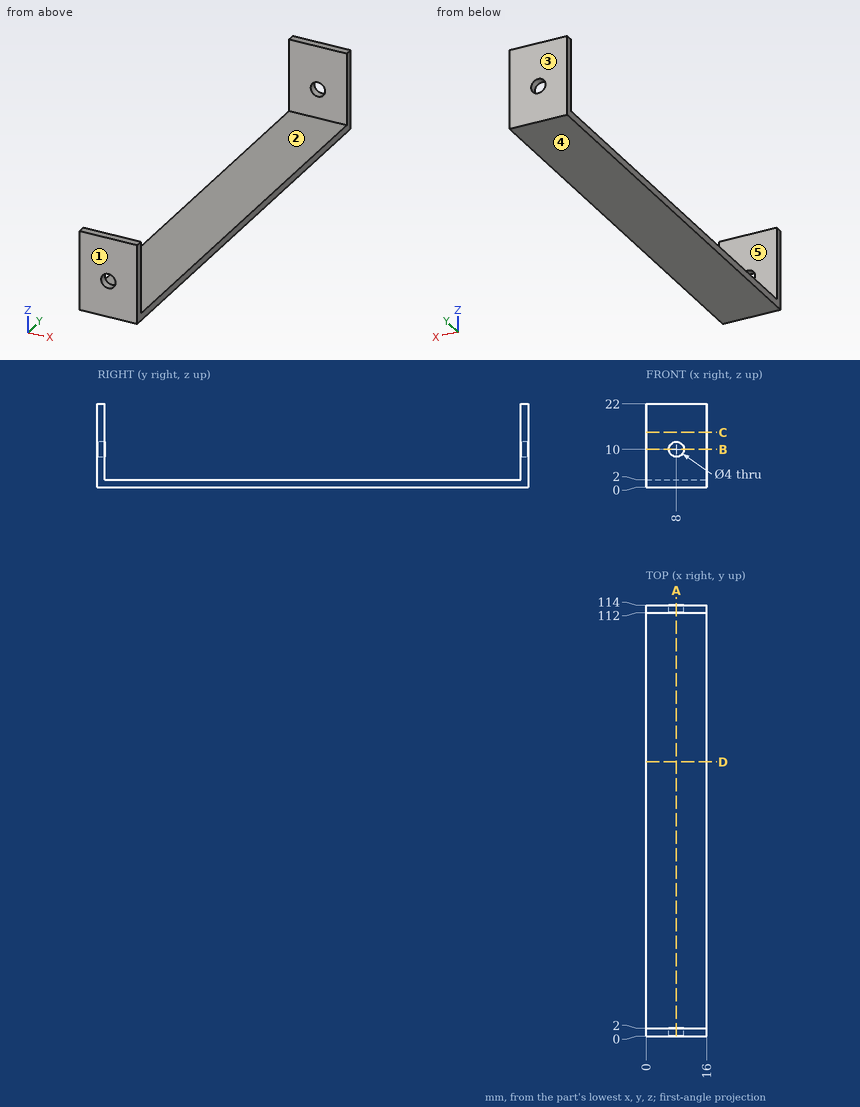
Can you work these out from the drawing? Everything is in mm from the part's minimum corner. A direction names the side the tool comes from. Coordinates: 2 decimals unless noted, no trailing zeros. Loops run counter-clockwise (first coordinate to the right, second up) from the corner with the lowest first, then second, coordinate; pieces in that order, holes last. Notation, with made-up numbers: M 1,46.25 L 7,46.25 A18 ccw 7,74.25 Z; hole C 70.25,-29.5 d10. An arc over 180 degrees is marked long. One line per item, written item: value.
1. Will this pin go through, and if not, where does the flat tip stop? pin 1 Ø1.5 at (x, y) = (8.5, 67.5) entering from +Z.
Geometry says:
pin 1: stops at z = 2
2. On a 3-axis mill with a long thin cutter (end or side, diameter ignored), from which of +Z, -Z, +X, -X, +Y, -Y can I reach the whole of each face in a straight line? I mean the marked faces 4 and 5. Say none if no direction works.
Geometry says:
face 4: -Z, +X, -X, +Y, -Y
face 5: +Z, +X, -X
3. Thinking about a two-plate mould opening in Y: for the marked faces 1, 2 and 3, which applies, +Y half, -Y half, draft (parallel to the pull), parting line (faces both ways), or undercut?
Geometry says:
face 1: -Y half
face 2: undercut
face 3: +Y half
4. Imagine slicing it at D-D (y = 72.5). List the corners of the cut face in (x, z) for me.
Geometry says:
outline: M 0,0 L 16,0 L 16,2 L 0,2 Z
5. Imagine slicing it at C-C (z = 14.5). List the corners of the cut face in (x, y) for me.
Geometry says:
outline: M 0,0 L 16,0 L 16,2 L 0,2 Z; M 0,112 L 16,112 L 16,114 L 0,114 Z
6. Please list where these lines run through material, in increasing order: probe 1 along X at (y, z) = (1.4, 10); probe 2 along Y at (x, z) = (13.5, 10); probe 3 along Z at (x, y) = (10.25, 55).
Geometry says:
probe 1: x = 0 to 6, 10 to 16
probe 2: y = 0 to 2, 112 to 114
probe 3: z = 0 to 2
7. Imagine slicing it at B-B (z = 10). List the corners of the cut face in (x, y) for me.
Geometry says:
outline: M 0,0 L 6,0 L 6,2 L 0,2 Z; M 0,112 L 6,112 L 6,114 L 0,114 Z; M 10,0 L 16,0 L 16,2 L 10,2 Z; M 10,112 L 16,112 L 16,114 L 10,114 Z
8. Imagine slicing it at A-A (x = 8). List the corners of the cut face in (y, z) for me.
Geometry says:
outline: M 0,0 L 114,0 L 114,8 L 112,8 L 112,2 L 2,2 L 2,8 L 0,8 Z; M 0,12 L 2,12 L 2,22 L 0,22 Z; M 112,12 L 114,12 L 114,22 L 112,22 Z
